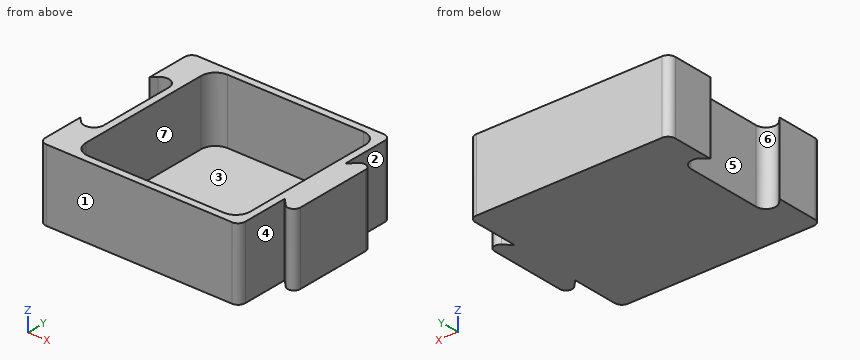
```python
from build123d import *

# Parameters (mm, degrees)
F0_W     = 63.5
F0_H     = 63.5
F1_DEPTH = 25.4
F2_T     = -2.54
F4_DEPTH = 25.4
F5_R     = 5.08
F6_R     = 2.54


with BuildPart() as f1:
    # F0 (on Top) → F1 (new body)
    with BuildSketch(Plane.XY):
        with Locations((31.75, 31.75)):
            Rectangle(F0_W, F0_H)
    extrude(amount=F1_DEPTH)

    # F2
    f2_openings = [f1.faces().sort_by_distance(p)[0] for p in [
        (31.75, 31.75, 25.4),
    ]]
    offset(amount=F2_T, openings=f2_openings)

    # F3 (on face) → F4 (join, through all)
    with BuildSketch(Plane.XY.offset(25.4)):
        with BuildLine():
            Line((66.0174359697, 46.9674359697), (63.5, 44.45))
            Line((63.5, 44.45), (63.5, 19.05))
            Line((63.5, 19.05), (66.0174359697, 16.5325640303))
            ThreePointArc((66.0174359697, 16.5325640303), (68.4640847787, 16.0458953235), (69.85, 18.1200640303))
            Line((69.85, 18.1200640303), (69.85, 45.3799359697))
            ThreePointArc((69.85, 45.3799359697), (68.4640847787, 47.4541046765), (66.0174359697, 46.9674359697))
        make_face()
        with BuildLine():
            Line((0, 45.3799359697), (0, 63.5))
            Line((0, 63.5), (-7.62, 63.5))
            Line((-7.62, 63.5), (-7.62, 46.2460512242))
            Line((-7.62, 46.2460512242), (-6.0005896424, 47.8654615818))
            ThreePointArc((-6.0005896424, 47.8654615818), (-2.1699072622, 48.6274316828), (0, 45.3799359697))
        make_face()
        with BuildLine():
            Line((-6.0005896424, 15.6345384182), (-7.62, 17.2539487758))
            Line((-7.62, 17.2539487758), (-7.62, 0))
            Line((-7.62, 0), (0, 0))
            Line((0, 0), (0, 18.1200640303))
            ThreePointArc((0, 18.1200640303), (-2.1699072622, 14.8725683172), (-6.0005896424, 15.6345384182))
        make_face()
    extrude(amount=-F4_DEPTH)

    # F5
    f5_edges = [f1.edges().sort_by_distance(p)[0] for p in [
        (2.54, 60.96, 13.97),
        (60.96, 60.96, 13.97),
        (2.54, 2.54, 13.97),
        (60.96, 2.54, 13.97),
    ]]
    fillet(f5_edges, radius=F5_R)

    # F6
    f6_edges = [f1.edges().sort_by_distance(p)[0] for p in [
        (-7.62, 63.5, 12.7),
        (63.5, 63.5, 12.7),
        (63.5, 0, 12.7),
        (-7.62, 0, 12.7),
    ]]
    fillet(f6_edges, radius=F6_R)


solid = f1.part
```
Build history of the part. All positions in model axes, mm. Face numbers are marked on the shaded views. A direction names the side the tool comes from. Give positions to 0.01 mm unless a question says otherwise; leave off trailing zeros. Loops run counter-clockwise (first coordinate to the right, second up) from the corner with the lowest first, then second, coordinate; pieces in that order, holes last. Notation, with made-up numbers: (36, 6.25) - (73, 6.25) arc R17 ccw to (73, 19.25) - close; hole circle Ø8 at (51, 86.25). An arc over 180 degrees is marked (long way). Use a Markdown table: item, result.
(1) Which spindle directions (+Z, -Z, +X, -X, +Y, -Y) get a long thin tool onto all of the face, cutting with end or side? Do the marked faces 4, 5, 6 and 7. Say none if no direction does.
Taken from the geometry:
| item | result |
|---|---|
| face 4 | +Z, -Z, -Y |
| face 5 | +Z, -Z, -X |
| face 6 | +Z, -Z |
| face 7 | +Z |
(2) Band-saw the part on A-A (z = 7.5). Give the cut face in (x, y).
Taken from the geometry:
| item | result |
|---|---|
| outline | (-7.62, 2.54) arc R2.54 ccw to (-5.08, 0) - (60.96, 0) arc R2.54 ccw to (63.5, 2.54) - (63.5, 19.05) - (66.02, 16.53) arc R2.25 ccw to (69.85, 18.12) - (69.85, 45.38) arc R2.25 ccw to (66.02, 46.97) - (63.5, 44.45) - (63.5, 60.96) arc R2.54 ccw to (60.96, 63.5) - (-5.08, 63.5) arc R2.54 ccw to (-7.62, 60.96) - (-7.62, 46.25) - (-6, 47.87) arc R3.52 cw to (0, 45.38) - (0, 18.12) arc R3.52 cw to (-6, 15.63) - (-7.62, 17.25) - close; hole (2.54, 7.62) arc R5.08 ccw to (7.62, 2.54) - (55.88, 2.54) arc R5.08 ccw to (60.96, 7.62) - (60.96, 55.88) arc R5.08 ccw to (55.88, 60.96) - (7.62, 60.96) arc R5.08 ccw to (2.54, 55.88) - close |
(3) Wall check: line 1 along Y through (x, z) = (42, 13); line 2 along X through (y, z) = (13.5, 15); line 3 along X through (y, z) = (15, 4.5). Give the ranges that are in metal, low to high.
Taken from the geometry:
| item | result |
|---|---|
| line 1 | 0 to 2.54, 60.96 to 63.5 |
| line 2 | -7.62 to 2.54, 60.96 to 63.5 |
| line 3 | -7.62 to -5.13, -1.9 to 2.54, 60.96 to 63.5 |
(4) Band-saw the part on B-B (x = 46.5). Give the cut face in (y, z).
Taken from the geometry:
| item | result |
|---|---|
| outline | (0, 0) - (63.5, 0) - (63.5, 25.4) - (60.96, 25.4) - (60.96, 2.54) - (2.54, 2.54) - (2.54, 25.4) - (0, 25.4) - close |
(5) Pull direction Y, two halves, no side cores. Call the marked faces 1, 2 and 3: +Y half, -Y half, draft (parallel to the pull), parting line (faces both ways), or undercut.
Taken from the geometry:
| item | result |
|---|---|
| face 1 | -Y half |
| face 2 | draft |
| face 3 | undercut |
(6) Band-saw the part on D-D (x = -1.5). Give the cut face in (y, z), and give its area (3 significant figures).
Taken from the geometry:
| item | result |
|---|---|
| outline | (0, 0) - (15.24, 0) - (15.24, 25.4) - (0, 25.4) - close; (48.26, 0) - (63.5, 0) - (63.5, 25.4) - (48.26, 25.4) - close |
| area | 774 mm2 |
(7) Band-saw the part on C-C (y = 54.5). Give the cut face in (x, z).
Taken from the geometry:
| item | result |
|---|---|
| outline | (-7.62, 0) - (63.5, 0) - (63.5, 25.4) - (60.96, 25.4) - (60.96, 2.54) - (2.54, 2.54) - (2.54, 25.4) - (-7.62, 25.4) - close |
(8) Drop flat-ended pins along their axis: pin 1 Ø12.5 at (y, z) = (26.5, 8.5) entering from -X; pin 2 Ø8.5 at (y, z) = (50, 14.5) entering from +X. Give the stop position or say it passes through.
Taken from the geometry:
| item | result |
|---|---|
| pin 1 | x = 0 |
| pin 2 | x = 69.82 |
